Can you work these out from the model? Positions are in its coordinate system, mm. Face numbers are marked on the shaded views. A direction names the side the tool comes from. Round coordinates to 2 decimals unless told otherwise and drop trailing zeros. Order: outer loops, then holes, each group sorted by start corner. A loop starts at its lowest first (then second) coordinate and runs counter-clockwise, first axis right, second up. Notation, with made-up numbers: M -17.5,4.25 L 20.5,4.25 A14 ccw 20.5,12.25 Z; hole C 12,61.5 d10. An arc over 180 degrees is marked long. Answer as CSV lines item,"result". Start each with the question number.
from build123d import *

# Parameters (mm, degrees)
BOSS_EXTRUDE1_DEPTH = 25
BOSS_EXTRUDE3_DEPTH = 20
SKETCH3_R           = 7
CUT_EXTRUDE1_DEPTH  = 20
SKETCH4_R           = 7
CUT_EXTRUDE2_DEPTH  = 20
BOSS_EXTRUDE4_REACH = 52
SKETCH5_W           = 40
SKETCH5_H           = 30
SKETCH6_W           = 30
SKETCH6_H           = 20
CUT_EXTRUDE3_DEPTH  = 10
CUT_EXTRUDE4_REACH  = 42
SKETCH7_R           = 7.5


with BuildPart() as part:
    # Sketch1 → Boss-Extrude1 (new body, symmetric)
    with BuildSketch(Plane.XY):
        with BuildLine():
            Line((-40, 0), (-35, 0))
            Line((-35, 0), (-35, 5))
            Line((-35, 5), (-29.580398915, 5))
            ThreePointArc((-29.580398915, 5), (0, 30), (29.580398915, 5))
            Line((29.580398915, 5), (35, 5))
            Line((35, 5), (35, 0))
            Line((35, 0), (40, 0))
            ThreePointArc((40, 0), (0, 40), (-40, 0))
        make_face()
    extrude(amount=BOSS_EXTRUDE1_DEPTH, both=True)

    # Sketch2 → Boss-Extrude3 (add)
    with BuildSketch(Plane(origin=(0, 0, 0), x_dir=(1, 0, 0), z_dir=(0, 1, 0))):
        with BuildLine():
            Line((35, 14.624040257), (35, -15.375959743))
            Line((35, -15.375959743), (55, -15.375959743))
            ThreePointArc((55, -15.375959743), (70, -0.375959743), (55, 14.624040257))
            Line((55, 14.624040257), (35, 14.624040257))
        make_face()
        with BuildLine():
            Line((-55, -15.375959743), (-35, -15.375959743))
            Line((-35, -15.375959743), (-35, 14.624040257))
            Line((-35, 14.624040257), (-55, 14.624040257))
            ThreePointArc((-55, 14.624040257), (-70, -0.375959743), (-55, -15.375959743))
        make_face()
    extrude(amount=BOSS_EXTRUDE3_DEPTH)

    # Sketch3 → Cut-Extrude1 (cut)
    with BuildSketch(Plane(origin=(0, 20, 0), x_dir=(1, 0, 0), z_dir=(0, 1, 0))):
        with Locations((55, -0.375959743)):
            Circle(SKETCH3_R)
    extrude(amount=-CUT_EXTRUDE1_DEPTH, mode=Mode.SUBTRACT)

    # Sketch4 → Cut-Extrude2 (cut)
    with BuildSketch(Plane(origin=(0, 20, 0), x_dir=(1, 0, 0), z_dir=(0, 1, 0))):
        with Locations((-55, -0.375959743)):
            Circle(SKETCH4_R)
    extrude(amount=-CUT_EXTRUDE2_DEPTH, mode=Mode.SUBTRACT)

    # Sketch5 → Boss-Extrude4 (add, up to next)
    with BuildSketch(Plane(origin=(0, 50, 0), x_dir=(1, 0, 0), z_dir=(0, 1, 0)), mode=Mode.PRIVATE) as boss_extrude4_sk1:
        Rectangle(SKETCH5_W, SKETCH5_H)
    boss_extrude4_tool1 = extrude(boss_extrude4_sk1.sketch, amount=-BOSS_EXTRUDE4_REACH, mode=Mode.PRIVATE) - part.part
    add(boss_extrude4_tool1.solids().sort_by_distance((0, 50, 0))[0])

    # Sketch6 → Cut-Extrude3 (cut)
    with BuildSketch(Plane(origin=(0, 50, 0), x_dir=(1, 0, 0), z_dir=(0, 1, 0))):
        Rectangle(SKETCH6_W, SKETCH6_H)
    extrude(amount=-CUT_EXTRUDE3_DEPTH, mode=Mode.SUBTRACT)

    # Sketch7 → Cut-Extrude4 (cut, up to next)
    with BuildSketch(Plane(origin=(0, 40, 0), x_dir=(1, 0, 0), z_dir=(0, 1, 0)), mode=Mode.PRIVATE) as cut_extrude4_sk1:
        Circle(SKETCH7_R)
    cut_extrude4_tool1 = extrude(cut_extrude4_sk1.sketch, amount=-CUT_EXTRUDE4_REACH, mode=Mode.PRIVATE) & part.part
    add(cut_extrude4_tool1.solids().sort_by_distance((0, 40, 0))[0], mode=Mode.SUBTRACT)


solid = part.part
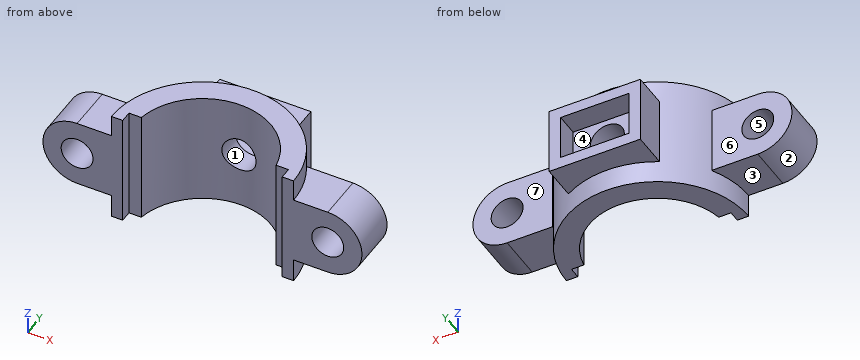
(1) I want a section at A-A on x = 0. Write out the boundary of the cut face in (y, z).
(2) If we mould it in two halves opening along X, with no side actions, what happens to the marked faces 1, 2 and 3? For each: +X half, -X half, draft (parallel to the pull), parting line (faces both ways), or undercut.
(3) I'm going to push flat-ended pins straight in: P1, Ø0.5, axis at y = 19.5, z = 4, coming from the -X side; P2, Ø2.5, axis at x = 32.5, z = -3, coming from the -Y side; P3, Ø1.5, axis at x = 41, z = -8.5, coming from the +Y side. Where does each tip first touch, or does it pass through?
(4) I want a section at C-C on z = -18. Write out the boundary of the cut face in (x, y), and give its area (3 significant figures).
(5) I want a section at D-D on y = 37. Write out the boundary of the cut face in (x, z), and give its area (3 significant figures).
(6) If I drill on line 1 along X through (y, z) = (35.5, 0); line 2 along Z through (x, y) = (55, 11.5); line 3 along Z through (x, y) = (-6, 40.5), over which ranges is the centre line in solid material (lowest first)?
(7) For the marked faces 4, 5, 6 and 7, which set-ups out of +Z, -Z, +X, -X, +Y, -Y let a thin tool reach every point of the face, with its end or its side?
(8) I want a section at B-B on y = 13. Write out the boundary of the cut face in (x, z), and give its area (3 significant figures).
From the geometry:
1,outline,"M 30,-25 L 40,-25 L 40,-15 L 50,-15 L 50,-10 L 40,-10 L 40,-7.5 L 30,-7.5 Z; M 30,7.5 L 40,7.5 L 40,10 L 50,10 L 50,15 L 40,15 L 40,25 L 30,25 Z"
2,face 1,"undercut"
2,face 2,"-X half"
2,face 3,"draft"
3,P1,"x = -69.62"
3,P2,"y = 5"
3,P3,"y = 20"
4,outline,"M -40,0 L -35,0 L -35,5 L -29.58,5 A30 cw 29.58,5 L 35,5 L 35,0 L 40,0 A40 ccw Z"
4,area,"1,050 mm²"
5,outline,"M -20,-15 L -15.2,-15 L -15.2,-25 L 15.2,-25 L 15.2,-15 L 20,-15 L 20,15 L 15.2,15 L 15.2,25 L -15.2,25 L -15.2,15 L -20,15 Z; hole C 0,0 d15"
5,area,"1,630 mm²"
6,line 1,"-20 to -7.5, 7.5 to 20"
6,line 2,"-14.62 to -6.62, 7.38 to 15.38"
6,line 3,"-15 to -10, 10 to 15"
7,face 4,"+Y"
7,face 5,"+Y, -Y"
7,face 6,"+Z, -Z, -X, +Y"
7,face 7,"+Z, -Z, +X, +Y"
8,outline,"M -55,-14.62 L -37.83,-14.62 L -37.83,-25 L -27.04,-25 L -27.04,25 L -37.83,25 L -37.83,15.38 L -55,15.38 A15 ccw Z; M 27.04,-25 L 37.83,-25 L 37.83,-14.62 L 55,-14.62 A15 ccw 55,15.38 L 37.83,15.38 L 37.83,25 L 27.04,25 Z; hole C -55,0.38 d14; hole C 55,0.38 d14"
8,area,"2,510 mm²"
